Geometry: final body of the model. Coordinates: model frame, mm. A direction names the side the tool comes from. Round coordinates to 2 decimals unless told otherwise and drop trailing zeros. Loops run counter-clockwise (first coordinate to the right, second up) from the corner with the lowest first, then second, coordinate; pieces in that order, holes last. Notation, with made-up numbers: (54.5, 29) - (106.5, 29) arc R34 ccw to (106.5, 59) - close; hole circle Ø8 at (71, -16). An arc over 180 degrees is marked (long way). Return JSON: item names as keys, results as strings. Group by question number.
1. First-contact query: pin 1 Ø1.5 at (x, z) = (11, -7) entering from -Y; pin 2 Ø13 at (x, y) = (11, 15) entering from -Z. Flat tips, straight axial feed; report the tip coordinate or a pass-through.
2. Set-up query: faces 4 (the face through (7.5, 9.7, -7.9)), 5 (the face through (20.19, 2.67, -3.38)), 6 (the face through (11, 26, -5)). Return all of +Z, -Z, +X, -X, +Y, -Y with unobstructed straight access to the full face (end or side cutting, diameter ignored); none if empty.
3. Section C-C on y = 4. Return loops of the section in (x, z), and give its area (3 significant figures).
4. Section D-D on x = 17. Return loops of the section in (y, z), and give its area (3 significant figures).
5. Material intervals for probe 1 along X at (y, z) = (2.15, -7); probe 2 along Y at (x, z) = (11, -8.75); probe 3 along Z at (x, y) = (11, 2.9), sorted ascending.
6. Draft query along X for faces 1 (the face through (8, 7, -10)), 2 (the face through (22, 13, -5)), 3 (the face through (12.745, 7.141, -8.965)). Return one class per face: +X half, -X half, draft (parallel to the pull), parting line (faces both ways), or undercut.
7. Section A-A on y = 15. Return loops of the section in (x, z).
8. Section B-B on x = 13. Return loops of the section in (y, z), and give its area (3 significant figures).
from build123d import *

# Parameters (mm, degrees)
SKETCH1_W                       = 22
SKETCH1_H                       = 10
BOSS_EXTRUDE1_DEPTH             = 26
SKETCH7_R                       = 5.7
CUT_EXTRUDE1_DEPTH              = 11
SKETCH9_R                       = 8.05
CUT_EXTRUDE3_DEPTH              = 2.1
M3X0_5_TAPPED_HOLE1_D           = 2.5
M3X0_5_TAPPED_HOLE1_DEPTH       = 5
M3X0_5_TAPPED_HOLE1_CSINK_D     = 3.05
M3X0_5_TAPPED_HOLE1_CSINK_ANGLE = 90
M3X0_5_TAPPED_HOLE1_TIP         = 0.751075774


with BuildPart() as part:
    # Sketch1 → Boss-Extrude1 (new body)
    with BuildSketch(Plane(origin=(0, 0, 0), x_dir=(1, 0, 0), z_dir=(0, 1, 0))):
        with Locations((11, 5)):
            Rectangle(SKETCH1_W, SKETCH1_H)
    extrude(amount=BOSS_EXTRUDE1_DEPTH)

    # Sketch7 → Cut-Extrude1 (cut, through all)
    with BuildSketch(Plane.XY):
        with Locations((11, 15)):
            Circle(SKETCH7_R)
    extrude(amount=-CUT_EXTRUDE1_DEPTH, mode=Mode.SUBTRACT)

    # Sketch9 → Cut-Extrude3 (cut)
    with BuildSketch(Plane(origin=(0, 0, -10), x_dir=(-1, 0, 0), z_dir=(0, 0, -1))):
        with Locations((-11, 15)):
            Circle(SKETCH9_R)
    extrude(amount=-CUT_EXTRUDE3_DEPTH, mode=Mode.SUBTRACT)

    # M3x0.5 Tapped Hole1
    with Locations(Plane(origin=(0, 0, 0), x_dir=(-1, 0, 0), z_dir=(0, -1, 0))):
        with Locations((-3, 3), (-19, 3), (-11, 7)):
            CounterSinkHole(M3X0_5_TAPPED_HOLE1_D / 2, M3X0_5_TAPPED_HOLE1_CSINK_D / 2, depth=M3X0_5_TAPPED_HOLE1_DEPTH, counter_sink_angle=M3X0_5_TAPPED_HOLE1_CSINK_ANGLE)
            with Locations((0, 0, -(M3X0_5_TAPPED_HOLE1_DEPTH + M3X0_5_TAPPED_HOLE1_TIP / 2))):  # 118° drill point
                Cone(0, M3X0_5_TAPPED_HOLE1_D / 2, M3X0_5_TAPPED_HOLE1_TIP, mode=Mode.SUBTRACT)


solid = part.part
Taken from the geometry:
{
 "1": {"pin 1": "y = 5.3", "pin 2": "z = -7.9"},
 "2": {"face 4": "-Z", "face 5": "-Y", "face 6": "+Z, -Z, +X, -X, +Y"},
 "3": {"outline": "(0, -10) - (22, -10) - (22, 0) - (0, 0) - close; hole circle Ø2.5 at (3, -3); hole circle Ø2.5 at (11, -7); hole circle Ø2.5 at (19, -3)", "area": "205 mm2"},
 "4": {"outline": "(0, -10) - (9.63, -10) - (9.63, -7.9) - (20.37, -7.9) - (20.37, -10) - (26, -10) - (26, 0) - (0, 0) - close", "area": "237 mm2"},
 "5": {"probe 1": "0 to 9.75, 12.25 to 22", "probe 2": "0 to 6.95, 23.05 to 26", "probe 3": "-10 to -8.25, -5.75 to 0"},
 "6": {"face 1": "draft", "face 2": "+X half", "face 3": "undercut"},
 "7": {"outline": "(0, -10) - (2.95, -10) - (2.95, -7.9) - (5.3, -7.9) - (5.3, 0) - (0, 0) - close; (16.7, -7.9) - (19.05, -7.9) - (19.05, -10) - (22, -10) - (22, 0) - (16.7, 0) - close"},
 "8": {"outline": "(0, -10) - (7.2, -10) - (7.2, -7.9) - (9.66, -7.9) - (9.66, 0) - (0, 0) - close; (20.34, -7.9) - (22.8, -7.9) - (22.8, -10) - (26, -10) - (26, 0) - (20.34, 0) - close", "area": "143 mm2"}
}
